from build123d import *

# Parameters (mm, degrees)
F1_DEPTH = 40.2336
F0_R     = 10.16
F2_DEPTH = 15.7734
F3_R     = 3.302


with BuildPart() as f1:
    # F0 (on Top) → F1 (new body)
    with BuildSketch(Plane.XY):
        with BuildLine():
            ThreePointArc((-45.510295, 28.126541), (-79.127942, 0), (-45.510295, -28.126541))
            ThreePointArc((-45.510295, -28.126541), (-28.636917, -18.336262), (-21.977942, 0))
            ThreePointArc((-21.977942, 0), (-28.636917, 18.336262), (-45.510295, 28.126541))
        make_face()
        with BuildLine():
            ThreePointArc((-64.000707, 4.826), (-50.552942, 14.2875), (-37.105177, 4.826))
            Line((-37.105177, 4.826), (-34.144542, 4.826))
            Line((-34.144542, 4.826), (-34.144542, -4.826))
            Line((-34.144542, -4.826), (-37.105177, -4.826))
            ThreePointArc((-37.105177, -4.826), (-50.552942, -14.2875), (-64.000707, -4.826))
            ThreePointArc((-64.000707, -4.826), (-64.840442, 0), (-64.000707, 4.826))
        make_face(mode=Mode.SUBTRACT)
    extrude(amount=F1_DEPTH)

    # F0 (on Top) → F2 (join)
    with BuildSketch(Plane.XY):
        with BuildLine():
            Line((-45.510295, -28.126541), (6.783823, -18.751028))
            ThreePointArc((6.783823, -18.751028), (-15.627942, 0), (6.783823, 18.751028))
            Line((6.783823, 18.751028), (-45.510295, 28.126541))
            ThreePointArc((-45.510295, 28.126541), (-28.636917, 18.336262), (-21.977942, 0))
            ThreePointArc((-21.977942, 0), (-28.636917, -18.336262), (-45.510295, -28.126541))
        make_face()
        with BuildLine():
            ThreePointArc((6.783823, 18.751028), (-15.627942, 0), (6.783823, -18.751028))
            ThreePointArc((6.783823, -18.751028), (18.032741, -12.224174), (22.472058, 0))
            ThreePointArc((22.472058, 0), (18.032741, 12.224175), (6.783823, 18.751028))
        make_face()
        with Locations((3.422058, 0)):
            Circle(F0_R, mode=Mode.SUBTRACT)
    extrude(amount=F2_DEPTH)

    # F3
    f3_edges = [f1.edges().sort_by_distance(p)[0] for p in [
        (-55.595589, 28.126541, 40.2336),
    ]]
    fillet(f3_edges, radius=F3_R)


solid = f1.part
Read the model definition and answer for the solid it produces. Units are mm, in the model's axes. A direction names the side the tool comes from. Coordinates: 2 decimals unless noted, no trailing zeros. Order: outer loops, then holes, each group sorted by start corner. A loop starts at its lowest first (then second) coordinate and runs counter-clockwise, first axis right, second up. Notation, with made-up numbers: (36.5, 23.25) -> (89.5, 23.25) arc R22 cw to (89.5, 44.25) -> close; hole circle Ø10 at (-32.5, -39). An arc over 180 degrees is marked (long way). Answer as a JSON object with one key per item and string values.
1) A tool of negligible diameter and unlimited length cuts with its end or side. For faces 1 (the face through (-40, -11, 40.234)), 2 (the face through (-34.145, 0, 20)), from which of +Z, -Z, +X, -X, +Y, -Y can it reach the whole face along a straight path? Write none if from no direction.
Model answer:
{"face 1": "+Z, +X, -X, +Y, -Y", "face 2": "+Z, -Z"}
2) The mould has two halves that part along X. Classify faces 3 (the face through (-4.066, 6.867, 7.776)), 4 (the face through (-18.997, 23.373, 7.776)), 5 (the face through (-29, 0, 0)): released by +X, released by -X, zero draft, split by the parting line, or undercut.
Model answer:
{"face 3": "undercut", "face 4": "released by +X", "face 5": "zero draft"}
3) A cutting plane is placed at D-D, the plane x = -17.5. Determine the outline of the cut face in (y, z).
Model answer:
{"outline": "(-23.1, 0) -> (23.1, 0) -> (23.1, 15.77) -> (-23.1, 15.77) -> close"}
4) A cutting plane is placed at B-B, the plane z = 12. State how many separate pieces and enclosed holes the cut face has, plus the area to 3 significant figures.
Model answer:
{"separate pieces": "1", "enclosed holes": "2", "area": "3,470 mm²"}
5) Each of these flat-tipped pins is pushed along its axis until it touches: pin 1 (0.9 mm diameter, centred on x = -35.5, z = 10.5, fed in from +Y); pin 2 (8 mm diameter, centred on y = -11, z = 22, fed in from +X); pin 3 (12 mm diameter, centred on x = -55.5, z = 29.5, fed in from -Y) (3 decimals); pin 4 (12 mm diameter, centred on x = 10.5, z = 18, fed in from +Y). Where does it stop, or does it pass through?
Model answer:
{"pin 1": "stops at y = 26.41", "pin 2": "stops at x = -22.85", "pin 3": "stops at y = -28.575", "pin 4": "stops at y = 19.08"}
6) Consider line 1 along Z through (x, y) = (-17, 5.5); line 2 along Y through (x, z) = (-50.5, 17); line 3 along Y through (x, z) = (-41, 17). Determine where each line is inside the solid, lowest interval first. Write a range as from..to.
Model answer:
{"line 1": "z = 0..15.77", "line 2": "y = -28.57..-14.29, 14.29..28.57", "line 3": "y = -26.93..-10.62, 10.62..26.93"}
